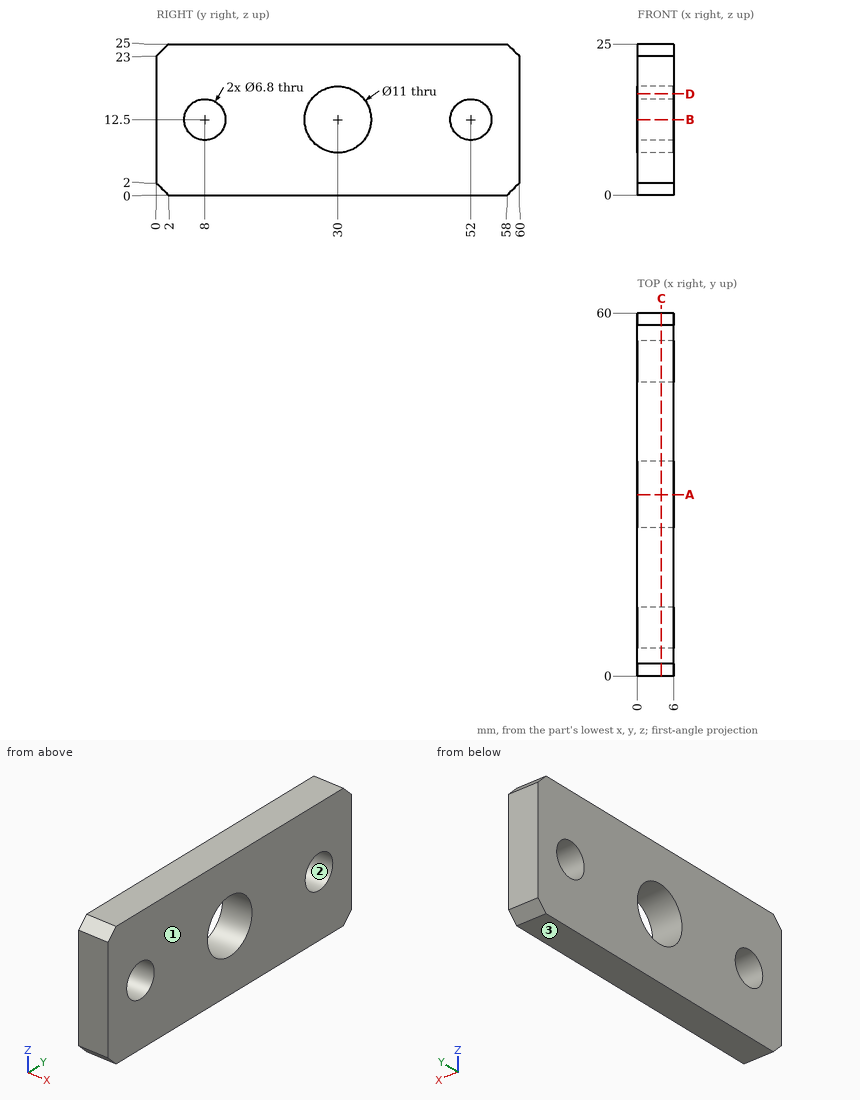
Study the drawing (mm; zero at the part's minimum x, y, z) and answer. Coordinates: 2 decimals unless noted, no trailing zeros. Loops run counter-clockwise (first coordinate to the right, second up) from the corner with the lowest first, then second, coordinate; pieces in that order, holes last. Notation, with made-up numbers: M 52,-19.75 L 61,-19.75 A9 cw 61,-3.75 Z; hole C -5.75,-13.5 d10. An arc over 180 degrees is marked long. Answer in a Markdown table with one row per item. Add a question column.
1. The mould has two halves that part along Z. Classify the marked faces 1, 2 and 3: pulls with the +Z half, pulls with the -Z half, needs draft (parallel to the pull), parting line crosses it, or undercut.
2. Find section B-B, the plane z = 12.5. Write down the section's boundary in (x, y), then the cut area to 3 significant figures.
3. Consider L1, parallel to Y at x = 3.85, z = 12.5; L2, parallel to Y at x = 2.85, z = 13.25; L3, parallel to Z at x = 4.25, y = 5. Determine where each line is inside the solid, lowest interval first.
4. Find section D-D, the plane z = 16.75. Write down the section's boundary in (x, y).
5. Find section C-C, the plane x = 4. Write down the section's boundary in (y, z).
6. Find section A-A, the plane y = 30. Write down the section's boundary in (x, z).
Reported:
| question | item | result |
|---|---|---|
| 1 | face 1 | needs draft |
| 1 | face 2 | undercut |
| 1 | face 3 | pulls with the -Z half |
| 2 | outline | M 0,0 L 6,0 L 6,4.6 L 0,4.6 Z; M 0,11.4 L 6,11.4 L 6,24.5 L 0,24.5 Z; M 0,35.5 L 6,35.5 L 6,48.6 L 0,48.6 Z; M 0,55.4 L 6,55.4 L 6,60 L 0,60 Z |
| 2 | area | 212 mm^2 |
| 3 | L1 | y = 0 to 4.6, 11.4 to 24.5, 35.5 to 48.6, 55.4 to 60 |
| 3 | L2 | y = 0 to 4.68, 11.32 to 24.55, 35.45 to 48.68, 55.32 to 60 |
| 3 | L3 | z = 0 to 10.9, 14.1 to 25 |
| 4 | outline | M 0,0 L 6,0 L 6,26.51 L 0,26.51 Z; M 0,33.49 L 6,33.49 L 6,60 L 0,60 Z |
| 5 | outline | M 0,2 L 2,0 L 58,0 L 60,2 L 60,23 L 58,25 L 2,25 L 0,23 Z; hole C 8,12.5 d6.8; hole C 30,12.5 d11; hole C 52,12.5 d6.8 |
| 6 | outline | M 0,0 L 6,0 L 6,7 L 0,7 Z; M 0,18 L 6,18 L 6,25 L 0,25 Z |
